```python
from build123d import *

# Parameters (mm, degrees)
SKETCH1_R           = 97.5
BOSS_EXTRUDE1_DEPTH = 30
SKETCH2_R           = 5
CUT_EXTRUDE1_DEPTH  = 142.111657917
SKETCH3_R           = 6.357711216
CUT_EXTRUDE2_DEPTH  = 23.505334
CIRPATTERN1_START   = 6.494666397
CIRPATTERN1_DEPTH   = 23.505333603


# Read off the part's stored shape, not the designer's step: CirPattern1
with BuildPart() as part:
    # Sketch1 → Boss-Extrude1 (new body)
    with BuildSketch(Plane(origin=(0, 0, 0), x_dir=(1, 0, 0), z_dir=(0, 1, 0))):
        with Locations(Location((0, 0, 0), (0, 0, 270))):
            Circle(SKETCH1_R)
    extrude(amount=BOSS_EXTRUDE1_DEPTH)

    # Sketch2 → Cut-Extrude1 (cut, through all)
    with BuildSketch(Plane(origin=(0, 0, 0), x_dir=(1, 0, 0), z_dir=(0, 1, 0))):
        with Locations(Location((0, 0, 0), (0, 0, 270))):
            Circle(SKETCH2_R)
    extrude(amount=CUT_EXTRUDE1_DEPTH, mode=Mode.SUBTRACT)

    # Sketch3 → Cut-Extrude2 (cut)
    with BuildSketch(Plane(origin=(0, 30, 0), x_dir=(1, 0, 0), z_dir=(0, 1, 0))):
        with Locations(Location((-15.425910616, 0, 0), (0, 0, 270))):
            Circle(SKETCH3_R)
    extrude(amount=-CUT_EXTRUDE2_DEPTH, mode=Mode.SUBTRACT)

    # CirPattern1 outline → CirPattern1 (cut)
    with BuildSketch(Plane(origin=(0, 0, 0), x_dir=(1, 0, 0), z_dir=(0, 1, 0)).offset(CIRPATTERN1_START)):
        with BuildLine():
            ThreePointArc((4.550535725, -10.985965062), (0, -9.0681994), (-4.550535725, -10.985965062))
            ThreePointArc((-4.550535725, -10.985965062), (-6.412185289, -6.412185289), (-10.985965062, -4.550535725))
            ThreePointArc((-10.985965062, -4.550535725), (-12.992919866, -5.873759266), (-15.347711556, -6.357230278))
            ThreePointArc((-15.347711556, -6.357230278), (-15.403346716, -15.403346716), (-6.357230278, -15.347711556))
            ThreePointArc((-6.357230278, -15.347711556), (0, -21.783621831), (6.357230278, -15.347711556))
            ThreePointArc((6.357230278, -15.347711556), (15.403346716, -15.403346716), (15.347711556, -6.357230278))
            ThreePointArc((15.347711556, -6.357230278), (21.783621831, 0), (15.347711556, 6.357230278))
            ThreePointArc((15.347711556, 6.357230278), (15.403346716, 15.403346716), (6.357230278, 15.347711556))
            ThreePointArc((6.357230278, 15.347711556), (0, 21.783621831), (-6.357230278, 15.347711556))
            ThreePointArc((-6.357230278, 15.347711556), (-15.403346716, 15.403346716), (-15.347711556, 6.357230278))
            ThreePointArc((-15.347711556, 6.357230278), (-12.992919866, 5.873759266), (-10.985965062, 4.550535725))
            ThreePointArc((-10.985965062, 4.550535725), (-6.412185289, 6.412185289), (-4.550535725, 10.985965062))
            ThreePointArc((-4.550535725, 10.985965062), (0, 9.0681994), (4.550535725, 10.985965062))
            ThreePointArc((4.550535725, 10.985965062), (6.412185289, 6.412185289), (10.985965062, 4.550535725))
            ThreePointArc((10.985965062, 4.550535725), (9.0681994, 0), (10.985965062, -4.550535725))
            ThreePointArc((10.985965062, -4.550535725), (6.412185289, -6.412185289), (4.550535725, -10.985965062))
        make_face()
    extrude(amount=CIRPATTERN1_DEPTH, mode=Mode.SUBTRACT)


solid = part.part
```
Geometry check sheet. Reference: the model listing, model coordinates, mm. A direction names the side the tool comes from. Round coordinates to 2 decimals unless told otherwise and drop trailing zeros. Loops run counter-clockwise (first coordinate to the right, second up) from the corner with the lowest first, then second, coordinate; pieces in that order, holes last. Notation, with made-up numbers: (-29, 6) -> (20, 6) arc R31 cw to (20, 34) -> close; hole circle Ø8 at (46, 71). An arc over 180 degrees is marked (long way). Use a Markdown table: item, result.
(1) Set-up check for faces 1 (the flat face through (11, 6.495, 0)), 2 (the flat face through (-20, 0, -1)): record each of +Z, -Z, +X, -X, +Y, -Y from which the full face is reachable in a straight line by a thin tool's end or side.
Calculated:
| item | result |
|---|---|
| face 1 | +Y |
| face 2 | +Z, -Z, +X, -X, -Y |
(2) Sectioned sample at C-C (x = 0). Enter the section's corners in (y, z).
Calculated:
| item | result |
|---|---|
| outline | (0, -97.5) -> (30, -97.5) -> (30, -21.78) -> (6.49, -21.78) -> (6.49, -9.07) -> (30, -9.07) -> (30, -5) -> (0, -5) -> close; (0, 5) -> (30, 5) -> (30, 9.07) -> (6.49, 9.07) -> (6.49, 21.78) -> (30, 21.78) -> (30, 97.5) -> (0, 97.5) -> close |
(3) Sectioned sample at B-B (y = 13.75). Enter the section's corners in (x, z), then the cut area to 3 significant figures.
Calculated:
| item | result |
|---|---|
| outline | circle Ø195 at (0, 0); (-10.99, -4.55) arc R6.36 cw to (-4.55, -10.99) arc R6.36 cw to (4.55, -10.99) arc R6.36 cw to (10.99, -4.55) arc R6.36 cw to (10.99, 4.55) arc R6.36 cw to (4.55, 10.99) arc R6.36 cw to (-4.55, 10.99) arc R6.36 cw to (-10.99, 4.55) arc R6.36 cw to start; hole (-15.35, -6.36) arc R6.36 ccw (long way) to (-6.36, -15.35) arc R6.36 ccw (long way) to (6.36, -15.35) arc R6.36 ccw (long way) to (15.35, -6.36) arc R6.36 ccw (long way) to (15.35, 6.36) arc R6.36 ccw (long way) to (6.36, 15.35) arc R6.36 ccw (long way) to (-6.36, 15.35) arc R6.36 ccw (long way) to (-15.35, 6.36) arc R6.36 ccw (long way) to start; hole circle Ø10 at (0, 0) |
| area | 28,800 mm² |
(4) Sectioned sample at D-D (z = 78). Enter the section's corners in (x, y).
Calculated:
| item | result |
|---|---|
| outline | (-58.5, 0) -> (58.5, 0) -> (58.5, 30) -> (-58.5, 30) -> close |
(5) Scan lines: probe 1 along Z at (x, y) = (12, 15.25); probe 2 along X at (y, z) = (2.5, 53); probe 3 along X at (y, z) = (15.5, -60). Record each from-to range of solid material in increasing order.
Calculated:
| item | result |
|---|---|
| probe 1 | -96.76 to -17.17, 17.17 to 96.76 |
| probe 2 | -81.84 to 81.84 |
| probe 3 | -76.85 to 76.85 |
(6) Go/stop test with flat-tipped pins: P1, Ø6, axis at x = -31.5, y = 21.5, coming from the +Z side; P2, Ø6, axis at y = 25, z = -51, coming from the +X side; P3, Ø5, axis at y = 6.5, z = 10, coming from the +X side. Record where each tip stops, or that it passes through.
Calculated:
| item | result |
|---|---|
| P1 | z = 93.24 |
| P2 | x = 84.87 |
| P3 | x = 97.21 |
(7) Mould release check, pull along X, two halves, no side actions. Record for faces 3 (the cylindrical face through (-6.362, 18.083, 6.463)), 4 (the cylindrical face through (-86.5, 14.79, 44.99)), 5 (the flat face through (1, 30, -23)): released by +X, released by -X, zero draft, split by the parting line, or undercut.
Calculated:
| item | result |
|---|---|
| face 3 | undercut |
| face 4 | split by the parting line |
| face 5 | zero draft |
(8) Sectioned sample at A-A (z = 0). Enter the section's corners in (x, y).
Calculated:
| item | result |
|---|---|
| outline | (-97.5, 0) -> (-5, 0) -> (-5, 30) -> (-9.07, 30) -> (-9.07, 6.49) -> (-21.78, 6.49) -> (-21.78, 30) -> (-97.5, 30) -> close; (5, 0) -> (97.5, 0) -> (97.5, 30) -> (21.78, 30) -> (21.78, 6.49) -> (9.07, 6.49) -> (9.07, 30) -> (5, 30) -> close |
